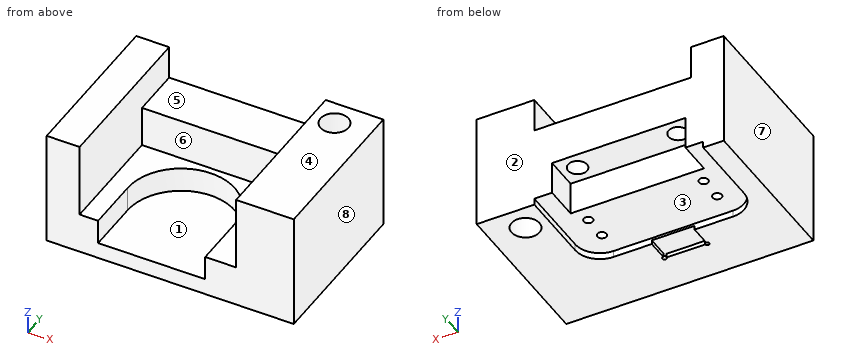
```python
from build123d import *

# Parameters (mm, degrees)
SKETCH_1_W           = 30
SKETCH_1_H           = 24
EXTRUDE_1_DEPTH      = 10
CUT_EXTRUDE_2_DEPTH  = 0.8
M1_4X0_3_2_D         = 1.1
M1_4X0_3_2_DEPTH     = 3.7
M1_4X0_3_2_TIP       = 0.33047334
CUT_EXTRUDE_4_DEPTH  = 0.5
SKETCH_12_W          = 30
SKETCH_12_H          = 4.25
CUT_EXTRUDE_5_DEPTH  = 10
SKETCH_13_R          = 1.7
CUT_EXTRUDE_6_DEPTH  = 10
SKETCH_14_W          = 23
SKETCH_14_H          = 19.75
CUT_EXTRUDE_7_DEPTH  = 5
CUT_EXTRUDE_9_DEPTH  = 3
SKETCH_20_W          = 7
SKETCH_20_H          = 19.75
SKETCH_20_R          = 1.7
EXTRUDE_3_DEPTH      = 4.1
SKETCH_23_W          = 4
SKETCH_23_H          = 19.75
EXTRUDE_4_DEPTH      = 9.1
SKETCH_24_W          = 16.2
SKETCH_24_H          = 4.1
CUT_EXTRUDE_10_DEPTH = 4
SKETCH_25_W          = 19
SKETCH_25_H          = 6
EXTRUDE_6_DEPTH      = 5
SKETCH_28_R          = 1.15
CUT_EXTRUDE_12_DEPTH = 2


with BuildPart() as part:
    # Sketch 1 → Extrude 1 (new body)
    with BuildSketch(Plane.XY):
        with Locations((7.449728974, 4.736434109)):
            Rectangle(SKETCH_1_W, SKETCH_1_H)
    extrude(amount=EXTRUDE_1_DEPTH)

    # Sketch 2 → Cut-Extrude 2 (cut)
    with BuildSketch(Plane(origin=(0, 0, 0), x_dir=(-1, 0, 0), z_dir=(0, 0, -1))):
        with BuildLine():
            Line((5.050271026, 16.736434109), (-15.449728974, 16.736434109))
            Line((-15.449728974, 16.736434109), (-15.449728974, 7.736434109))
            ThreePointArc((-15.449728974, 7.736434109), (-14.571049317, 5.615113765), (-12.449728974, 4.736434109))
            Line((-12.449728974, 4.736434109), (2.050271026, 4.736434109))
            ThreePointArc((2.050271026, 4.736434109), (4.17159137, 5.615113765), (5.050271026, 7.736434109))
            Line((5.050271026, 7.736434109), (5.050271026, 16.736434109))
        make_face()
    extrude(amount=-CUT_EXTRUDE_2_DEPTH, mode=Mode.SUBTRACT)

    # M1.4x0.3 _2
    with Locations(Plane(origin=(0, 0, 0.8), x_dir=(-1, 0, 0), z_dir=(0, 0, -1))):
        with Locations((-12.199728974, 10.736434109), (1.800271026, 10.736434109), (-12.199728974, 7.736434109), (1.800271026, 7.736434109)):
            Hole(M1_4X0_3_2_D / 2, depth=M1_4X0_3_2_DEPTH)
            with Locations((0, 0, -(M1_4X0_3_2_DEPTH + M1_4X0_3_2_TIP / 2))):  # 118° drill point
                Cone(0, M1_4X0_3_2_D / 2, M1_4X0_3_2_TIP, mode=Mode.SUBTRACT)

    # Sketch 11 → Cut-Extrude 4 (cut)
    with BuildSketch(Plane(origin=(0, 0, 0), x_dir=(-1, 0, 0), z_dir=(0, 0, -1))):
        with BuildLine():
            Line((-7.549728974, 1.936434109), (-2.849728974, 1.936434109))
            ThreePointArc((-2.849728974, 1.936434109), (-2.422952278, 1.759657413), (-2.599728974, 2.186434109))
            Line((-2.599728974, 2.186434109), (-2.599728974, 4.736434109))
            Line((-2.599728974, 4.736434109), (-7.799728974, 4.736434109))
            Line((-7.799728974, 4.736434109), (-7.799728974, 2.186434109))
            ThreePointArc((-7.799728974, 2.186434109), (-7.976505669, 1.759657413), (-7.549728974, 1.936434109))
        make_face()
    extrude(amount=-CUT_EXTRUDE_4_DEPTH, mode=Mode.SUBTRACT)

    # Sketch 12 → Cut-Extrude 5 (cut)
    with BuildSketch(Plane(origin=(0, 0, 0), x_dir=(-1, 0, 0), z_dir=(0, 0, -1))):
        with Locations((-7.449728974, -5.138565891)):
            Rectangle(SKETCH_12_W, SKETCH_12_H)
    extrude(amount=-CUT_EXTRUDE_5_DEPTH, mode=Mode.SUBTRACT)

    # Sketch 13 → Cut-Extrude 6 (cut)
    with BuildSketch(Plane(origin=(0, 0, 0), x_dir=(-1, 0, 0), z_dir=(0, 0, -1))):
        with Locations((-18.199728974, 13.686434109)):
            Circle(SKETCH_13_R)
    extrude(amount=-CUT_EXTRUDE_6_DEPTH, mode=Mode.SUBTRACT)

    # Sketch 14 → Cut-Extrude 7 (cut)
    with BuildSketch(Plane.XY.offset(10)):
        with Locations((3.949728974, 6.861434109)):
            Rectangle(SKETCH_14_W, SKETCH_14_H)
    extrude(amount=-CUT_EXTRUDE_7_DEPTH, mode=Mode.SUBTRACT)

    # Sketch 16 → Cut-Extrude 9 (cut)
    with BuildSketch(Plane.XY.offset(5)):
        with BuildLine():
            Line((-1.300271026, -3.013565891), (11.699728974, -3.013565891))
            Line((11.699728974, -3.013565891), (11.699728974, 3.486434109))
            ThreePointArc((11.699728974, 3.486434109), (5.199728974, 9.986434109), (-1.300271026, 3.486434109))
            Line((-1.300271026, 3.486434109), (-1.300271026, -3.013565891))
        make_face()
    extrude(amount=-CUT_EXTRUDE_9_DEPTH, mode=Mode.SUBTRACT)

    # Sketch 20 → Extrude 3 (add)
    with BuildSketch(Plane.XY.offset(10)):
        with Locations((18.949728974, 6.861434109)):
            Rectangle(SKETCH_20_W, SKETCH_20_H)
        with Locations(Location((18.199728974, 13.686434109, 0), (0, 0, 180))):
            Circle(SKETCH_20_R, mode=Mode.SUBTRACT)
    extrude(amount=EXTRUDE_3_DEPTH)

    # Sketch 23 → Extrude 4 (add)
    with BuildSketch(Plane.XY.offset(5)):
        with Locations((-5.550271026, 6.861434109)):
            Rectangle(SKETCH_23_W, SKETCH_23_H)
    extrude(amount=EXTRUDE_4_DEPTH)

    # Sketch 24 → Cut-Extrude 10 (cut)
    with BuildSketch(Plane(origin=(0, 0, 0.8), x_dir=(-1, 0, 0), z_dir=(0, 0, -1))):
        with Locations((-5.199728974, 14.686434109)):
            Rectangle(SKETCH_24_W, SKETCH_24_H)
    extrude(amount=-CUT_EXTRUDE_10_DEPTH, mode=Mode.SUBTRACT)

    # Sketch 25 → Extrude 6 (add)
    with BuildSketch(Plane.XY.offset(5)):
        with Locations((5.949728974, 13.736434109)):
            Rectangle(SKETCH_25_W, SKETCH_25_H)
    extrude(amount=EXTRUDE_6_DEPTH)

    # Sketch 28 → Cut-Extrude 12 (cut)
    with BuildSketch(Plane(origin=(0, 0, 4.8), x_dir=(-1, 0, 0), z_dir=(0, 0, -1))):
        with Locations((-11.299728974, 14.736434109)):
            Circle(SKETCH_28_R)
        with Locations((0.900271026, 14.736434109)):
            Circle(SKETCH_28_R)
    extrude(amount=-CUT_EXTRUDE_12_DEPTH, mode=Mode.SUBTRACT)


solid = part.part
```
Input: part model. Units: mm. Frame: model coordinates. Face numbers are marked on the shaded views. A direction names the side the tool comes from. Coordinates: 2 decimals unless noted, no trailing zeros. Order: outer loops, then holes, each group sorted by start corner. A loop starts at its lowest first (then second) coordinate and runs counter-clockwise, first axis right, second up. Notation, with made-up numbers: (-38.5, 54.5) - (-14.5, 54.5) arc R23 ccw to (-14.5, 83.5) - close; hole circle Ø1 at (39.5, 65.5). An arc over 180 degrees is marked (long way). Return JSON: item names as keys, results as strings.
Q1. Draft query along X for the marked faces 6, 7 and 8. Return one class per face: +X half, -X half, draft (parallel to the pull), parting line (faces both ways), or undercut.
The answers:
{"face 6": "undercut", "face 7": "-X half", "face 8": "+X half"}
Q2. First-contact query: pin 1 (1.2 mm diameter, centred on x = 6, z = 3, fed in from +Y); pin 2 (0.9 mm diameter, centred on x = -1.8, y = 7.74, fed in from -Z); pin 3 (6 mm diameter, centred on x = 5, z = 11, fed in from -Y). Flat tips, straight axial feed; report the tip coordinate or a pass-through.
The answers:
{"pin 1": "stops at y = 12.64", "pin 2": "stops at z = 4.56", "pin 3": "stops at y = 10.74"}
Q3. Cut plane C-C (z = 6.25). Return loops of the section in (x, y), then the cut area to 3 significant figures.
The answers:
{"outline": "(-7.55, -3.01) - (-3.55, -3.01) - (-3.55, 10.74) - (15.45, 10.74) - (15.45, -3.01) - (22.45, -3.01) - (22.45, 16.74) - (-7.55, 16.74) - close; hole circle Ø2.3 at (-0.9, 14.74); hole circle Ø2.3 at (11.3, 14.74); hole circle Ø3.4 at (18.2, 13.69)", "area": "314 mm2"}
Q4. Cut plane B-B (z = 13.25). Return loops of the section in (x, y).
The answers:
{"outline": "(-7.55, -3.01) - (-3.55, -3.01) - (-3.55, 16.74) - (-7.55, 16.74) - close; (15.45, -3.01) - (22.45, -3.01) - (22.45, 16.74) - (15.45, 16.74) - close; hole circle Ø3.4 at (18.2, 13.69)"}
Q5. Cut plane D-D (x = 6.5). Return loops of the section in (y, z).
The answers:
{"outline": "(-3.01, 0) - (1.94, 0) - (1.94, 0.5) - (4.74, 0.5) - (4.74, 0.8) - (12.64, 0.8) - (12.64, 4.8) - (16.74, 4.8) - (16.74, 10) - (10.74, 10) - (10.74, 5) - (9.86, 5) - (9.86, 2) - (-3.01, 2) - close"}
Q6. Access query for the marked faces 1, 2, 3, 4 and 5. Directions: +Z, -Z, +X, -X, +Y, -Y. A direction counts if a zero-diameter tool reaches every point of the face in a straight line with its end or side. Return the directions, or none.
The answers:
{"face 1": "+Z, -Y", "face 2": "+Z, -Z, +X, -X, +Y", "face 3": "-Z, +Y", "face 4": "+Z, +X, -X, +Y, -Y", "face 5": "+Z, +Y, -Y"}
Q7. Cut plane A-A (y = -1). Return loops of the section in (x, z).
The answers:
{"outline": "(-7.55, 0) - (22.45, 0) - (22.45, 14.1) - (15.45, 14.1) - (15.45, 5) - (11.7, 5) - (11.7, 2) - (-1.3, 2) - (-1.3, 5) - (-3.55, 5) - (-3.55, 14.1) - (-7.55, 14.1) - close"}
Q8. Ray query, probe 1 along X at (y, z) = (2.75, 7); probe 2 along X at (y, z) = (15.5, 2.25); probe 3 along X at (y, z) = (14, 12.75). Return the intervals inside material, ascending.
The answers:
{"probe 1": "x = -7.55 to -3.55, 15.45 to 22.45", "probe 2": "x = -7.55 to -2.9, 13.3 to 22.45", "probe 3": "x = -7.55 to -3.55, 15.45 to 16.53, 19.87 to 22.45"}
